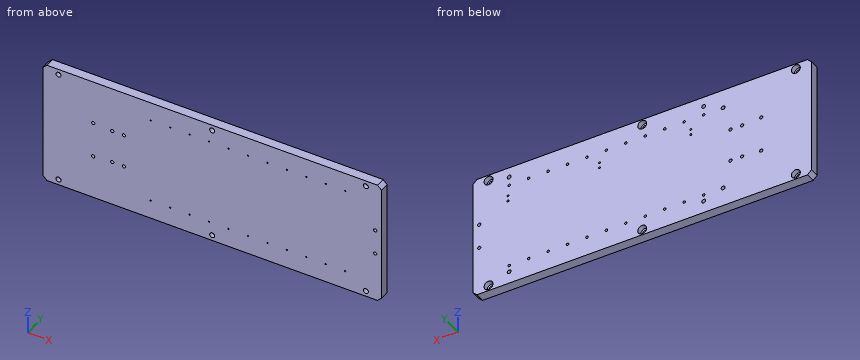
```python
from build123d import *

# Parameters (mm, degrees)
SKETCH_1_W                   = 435
SKETCH_1_H                   = 159.5
EXTRUDE_1_DEPTH              = 12
HOLE_WIZARD_M5_2_D           = 4.2
HOLE_WIZARD_M5_2_DEPTH       = 14
HOLE_WIZARD_M5_2_TIP         = 1.2618073
HOLE_WIZARD_M4_1_AT_2_COUNT  = 2
HOLE_WIZARD_M4_1_AT_2_PITCH  = 111
PATTERN_LINEAR_1_COUNT       = 11
PATTERN_LINEAR_1_PITCH       = 25
HOLE_WIZARD_M6_1_D           = 6.5
HOLE_WIZARD_M6_1_CBORE_D     = 11.5
HOLE_WIZARD_M6_1_CBORE_DEPTH = 6.5
CHAMFER_1_SIZE               = 5
HOLE_WIZARD_M3_1_AT_2_COUNT  = 2
HOLE_WIZARD_M3_1_AT_2_PITCH  = 7
PATTERN_LINEAR_2_COUNT       = 3
PATTERN_LINEAR_2_PITCH       = 117.5
HOLE_WIZARD_5_0_5_2_D        = 5
HOLE_WIZARD_5_0_5_2_DEPTH    = 10
HOLE_WIZARD_5_0_5_2_TIP      = 1.502151548


with BuildPart() as part:
    # Sketch 1 → Extrude 1 (new body)
    with BuildSketch(Plane(origin=(0, 0, 0), x_dir=(1, 0, 0), z_dir=(0, 1, 0))):
        with Locations((217.5, -79.75)):
            Rectangle(SKETCH_1_W, SKETCH_1_H)
    extrude(amount=EXTRUDE_1_DEPTH)

    # Hole Wizard M5 _2
    with Locations(Plane(origin=(0, 12, 0), x_dir=(1, 0, 0), z_dir=(0, 1, 0))):
        with Locations((64.5, -102.75), (64.5, -56.75), (89, -58.25), (104, -58.25), (89, -101.25), (104, -101.25), (427, -63.75), (427, -95.75)):
            Hole(HOLE_WIZARD_M5_2_D / 2, depth=HOLE_WIZARD_M5_2_DEPTH)
            with Locations((0, 0, -(HOLE_WIZARD_M5_2_DEPTH + HOLE_WIZARD_M5_2_TIP / 2))):  # 118° drill point
                Cone(0, HOLE_WIZARD_M5_2_D / 2, HOLE_WIZARD_M5_2_TIP, mode=Mode.SUBTRACT)

    # Sketch 6 → Hole Wizard M4 _1 (revolve, cut)
    with BuildSketch(Plane(origin=(388.5, 12, 24.25), x_dir=(0, 0, 1), z_dir=(1, 0, 0))):
        Polygon((0, 0), (0, 12.491420021), (1.65, 11.5), (1.65, 0), align=None)
    hole_wizard_m4_1 = revolve(axis=Axis((388.5, 18.35, 24.25), (0, -1, 0)), mode=Mode.SUBTRACT)

    # Hole Wizard M4 _1 at 2: Hole Wizard M4 _1 ×2
    with Locations(*[(0, 0, i * HOLE_WIZARD_M4_1_AT_2_PITCH) for i in range(1, HOLE_WIZARD_M4_1_AT_2_COUNT)]):
        add(hole_wizard_m4_1, mode=Mode.SUBTRACT)

    # Pattern Linear 1: Hole Wizard M4 _1 ×11
    with Locations(*[(-i * PATTERN_LINEAR_1_PITCH, 0, 0) for i in range(1, PATTERN_LINEAR_1_COUNT)]):
        add(hole_wizard_m4_1, mode=Mode.SUBTRACT)

    # Pattern Linear 1 copy 1 sketch → Pattern Linear 1 copy 1 (revolve, cut)
    with BuildSketch(Plane(origin=(363.5, 12, 135.25), x_dir=(0, 0, 1), z_dir=(1, 0, 0))):
        Polygon((0, 0), (0, 12.491420021), (1.65, 11.5), (1.65, 0), align=None)
    revolve(axis=Axis((363.5, 18.35, 135.25), (0, -1, 0)), mode=Mode.SUBTRACT)

    # Pattern Linear 1 copy 2 sketch → Pattern Linear 1 copy 2 (revolve, cut)
    with BuildSketch(Plane(origin=(338.5, 12, 135.25), x_dir=(0, 0, 1), z_dir=(1, 0, 0))):
        Polygon((0, 0), (0, 12.491420021), (1.65, 11.5), (1.65, 0), align=None)
    revolve(axis=Axis((338.5, 18.35, 135.25), (0, -1, 0)), mode=Mode.SUBTRACT)

    # Pattern Linear 1 copy 3 sketch → Pattern Linear 1 copy 3 (revolve, cut)
    with BuildSketch(Plane(origin=(313.5, 12, 135.25), x_dir=(0, 0, 1), z_dir=(1, 0, 0))):
        Polygon((0, 0), (0, 12.491420021), (1.65, 11.5), (1.65, 0), align=None)
    revolve(axis=Axis((313.5, 18.35, 135.25), (0, -1, 0)), mode=Mode.SUBTRACT)

    # Pattern Linear 1 copy 4 sketch → Pattern Linear 1 copy 4 (revolve, cut)
    with BuildSketch(Plane(origin=(288.5, 12, 135.25), x_dir=(0, 0, 1), z_dir=(1, 0, 0))):
        Polygon((0, 0), (0, 12.491420021), (1.65, 11.5), (1.65, 0), align=None)
    revolve(axis=Axis((288.5, 18.35, 135.25), (0, -1, 0)), mode=Mode.SUBTRACT)

    # Pattern Linear 1 copy 5 sketch → Pattern Linear 1 copy 5 (revolve, cut)
    with BuildSketch(Plane(origin=(263.5, 12, 135.25), x_dir=(0, 0, 1), z_dir=(1, 0, 0))):
        Polygon((0, 0), (0, 12.491420021), (1.65, 11.5), (1.65, 0), align=None)
    revolve(axis=Axis((263.5, 18.35, 135.25), (0, -1, 0)), mode=Mode.SUBTRACT)

    # Pattern Linear 1 copy 6 sketch → Pattern Linear 1 copy 6 (revolve, cut)
    with BuildSketch(Plane(origin=(238.5, 12, 135.25), x_dir=(0, 0, 1), z_dir=(1, 0, 0))):
        Polygon((0, 0), (0, 12.491420021), (1.65, 11.5), (1.65, 0), align=None)
    revolve(axis=Axis((238.5, 18.35, 135.25), (0, -1, 0)), mode=Mode.SUBTRACT)

    # Pattern Linear 1 copy 7 sketch → Pattern Linear 1 copy 7 (revolve, cut)
    with BuildSketch(Plane(origin=(213.5, 12, 135.25), x_dir=(0, 0, 1), z_dir=(1, 0, 0))):
        Polygon((0, 0), (0, 12.491420021), (1.65, 11.5), (1.65, 0), align=None)
    revolve(axis=Axis((213.5, 18.35, 135.25), (0, -1, 0)), mode=Mode.SUBTRACT)

    # Pattern Linear 1 copy 8 sketch → Pattern Linear 1 copy 8 (revolve, cut)
    with BuildSketch(Plane(origin=(188.5, 12, 135.25), x_dir=(0, 0, 1), z_dir=(1, 0, 0))):
        Polygon((0, 0), (0, 12.491420021), (1.65, 11.5), (1.65, 0), align=None)
    revolve(axis=Axis((188.5, 18.35, 135.25), (0, -1, 0)), mode=Mode.SUBTRACT)

    # Pattern Linear 1 copy 9 sketch → Pattern Linear 1 copy 9 (revolve, cut)
    with BuildSketch(Plane(origin=(163.5, 12, 135.25), x_dir=(0, 0, 1), z_dir=(1, 0, 0))):
        Polygon((0, 0), (0, 12.491420021), (1.65, 11.5), (1.65, 0), align=None)
    revolve(axis=Axis((163.5, 18.35, 135.25), (0, -1, 0)), mode=Mode.SUBTRACT)

    # Pattern Linear 1 copy 10 sketch → Pattern Linear 1 copy 10 (revolve, cut)
    with BuildSketch(Plane(origin=(138.5, 12, 135.25), x_dir=(0, 0, 1), z_dir=(1, 0, 0))):
        Polygon((0, 0), (0, 12.491420021), (1.65, 11.5), (1.65, 0), align=None)
    revolve(axis=Axis((138.5, 18.35, 135.25), (0, -1, 0)), mode=Mode.SUBTRACT)

    # Hole Wizard M6 _1 (through all)
    with Locations(Plane(origin=(0, 12, 0), x_dir=(1, 0, 0), z_dir=(0, 1, 0))):
        with Locations((20, -7.25), (217.5, -7.25), (415, -7.25), (20, -152.25), (217.5, -152.25), (415, -152.25)):
            CounterBoreHole(HOLE_WIZARD_M6_1_D / 2, HOLE_WIZARD_M6_1_CBORE_D / 2, HOLE_WIZARD_M6_1_CBORE_DEPTH)

    # Chamfer 1
    chamfer_1_edges = [part.edges().sort_by_distance(p)[0] for p in [
        (0, 6, 0),
        (435, 6, 0),
        (435, 6, 159.5),
        (0, 6, 159.5),
    ]]
    chamfer(chamfer_1_edges, length=CHAMFER_1_SIZE)

    # Sketch 10 → Hole Wizard M3 _1 (revolve, cut)
    with BuildSketch(Plane(origin=(155, 12, 121.25), x_dir=(0, 0, 1), z_dir=(1, 0, 0))):
        Polygon((0, 0), (0, 9.251075774), (1.25, 8.5), (1.25, 0), align=None)
    hole_wizard_m3_1 = revolve(axis=Axis((155, 18.35, 121.25), (0, -1, 0)), mode=Mode.SUBTRACT)

    # Hole Wizard M3 _1 at 2: Hole Wizard M3 _1 ×2
    with Locations(*[(0, 0, -i * HOLE_WIZARD_M3_1_AT_2_PITCH) for i in range(1, HOLE_WIZARD_M3_1_AT_2_COUNT)]):
        add(hole_wizard_m3_1, mode=Mode.SUBTRACT)

    # Pattern Linear 2: Hole Wizard M3 _1 ×3
    with Locations(*[(i * PATTERN_LINEAR_2_PITCH, 0, 0) for i in range(1, PATTERN_LINEAR_2_COUNT)]):
        add(hole_wizard_m3_1, mode=Mode.SUBTRACT)

    # Pattern Linear 2 copy 1 sketch → Pattern Linear 2 copy 1 (revolve, cut)
    with BuildSketch(Plane(origin=(272.5, 12, 114.25), x_dir=(0, 0, 1), z_dir=(1, 0, 0))):
        Polygon((0, 0), (0, 9.251075774), (1.25, 8.5), (1.25, 0), align=None)
    revolve(axis=Axis((272.5, 18.35, 114.25), (0, -1, 0)), mode=Mode.SUBTRACT)

    # Pattern Linear 2 copy 2 sketch → Pattern Linear 2 copy 2 (revolve, cut)
    with BuildSketch(Plane(origin=(390, 12, 114.25), x_dir=(0, 0, 1), z_dir=(1, 0, 0))):
        Polygon((0, 0), (0, 9.251075774), (1.25, 8.5), (1.25, 0), align=None)
    revolve(axis=Axis((390, 18.35, 114.25), (0, -1, 0)), mode=Mode.SUBTRACT)

    # Hole Wizard 5.0 _5_ _2
    with Locations(Plane(origin=(0, 12, 0), x_dir=(1, 0, 0), z_dir=(0, 1, 0))):
        with Locations((113.5, -135.25), (138.5, -146.75), (388.5, -146.75), (388.5, -15.75), (113.5, -24.25), (138.5, -15.75)):
            Hole(HOLE_WIZARD_5_0_5_2_D / 2, depth=HOLE_WIZARD_5_0_5_2_DEPTH)
            with Locations((0, 0, -(HOLE_WIZARD_5_0_5_2_DEPTH + HOLE_WIZARD_5_0_5_2_TIP / 2))):  # 118° drill point
                Cone(0, HOLE_WIZARD_5_0_5_2_D / 2, HOLE_WIZARD_5_0_5_2_TIP, mode=Mode.SUBTRACT)


solid = part.part
```
The listing builds one solid part. Answer for the finished solid, in the listing's coordinates (mm). Give positions to 0.01 mm unless a question says otherwise; leave off trailing zeros. Return JSON: item names as keys, results as strings. Group by question number.
1. Straight lines are drawn through the part: line 1 (X direction, y = 7.5, z = 152.25); line 2 (Z direction, x = 163.5, y = 3); line 3 (Z direction, x = 89, y = 4.25). For each, find the intervals that lie inside material, in ascending order. Write a range as [from, to].
2. Find section A-A (y = 7.5). State how many separate pieces and enclosed holes the cut face has, then the cut area to 3 significant figures.
3. Given pin 1 Ø6 at (x, z) = (416.5, 5.5) entering from +Y; pin 2 Ø4.5 at (x, z) = (288.5, 24.25) entering from +Y; pin 3 Ø3 at (x, z) = (363.5, 24.25) entering from +Y; pin 4 Ø2.5 at (x, z) = (138.5, 135.25) entering from +Y, each flat-ended and moving along its own axis, determine where each tip first touches the part or whether it passes through.
Verdict:
{
 "1": {"line 1": "x = [0, 14.25], [25.75, 211.75], [223.25, 409.25], [420.75, 435]", "line 2": "z = [0, 22.6], [25.9, 133.6], [136.9, 159.5]", "line 3": "z = [0, 56.15], [60.35, 99.15], [103.35, 159.5]"},
 "2": {"separate pieces": "1", "enclosed holes": "48", "area": "68,300 mm^2"},
 "3": {"pin 1": "stops at y = 5.5", "pin 2": "stops at y = 12", "pin 3": "stops at y = 0.41", "pin 4": "stops at y = 0.26"}
}
